from build123d import *

# Parameters (mm, degrees)
EXTRUDE_1_DEPTH        = 5
EXTRUDE_2_DEPTH        = 5
SKETCH_5_R             = 2.15
CUT_EXTRUDE_3_DEPTH    = 3.5
CUT_EXTRUDE_4_DEPTH    = 5
SKETCH_8_R             = 1.5
CUT_EXTRUDE_5_DEPTH    = 5
FILLET_1_R             = 2
FILLET_2_R             = 0.4
FILLET_4_R             = 2
FILLET_1_OF_MIRROR_2_R = 2
FILLET_2_OF_MIRROR_2_R = 0.4
FILLET_4_OF_MIRROR_2_R = 2
FILLET_3_R             = 2
SKETCH_10_R            = 0.8
CUT_EXTRUDE_6_DEPTH    = 10


with BuildPart() as part:
    # 草图2 → 凸台-拉伸1 (new body)
    with BuildSketch(Plane(origin=(0, 0, 0), x_dir=(1, 0, 0), z_dir=(0, 1, 0))):
        Polygon((0, -7.5), (0, 7.5), (-10.392304845, 13.5), (-18.392304845, 13.5), (-23.898712869, 11.116835995), (-104.216362147, 40.350069618), (-106.3513241, 34.484309861), (-103.323886643, 32.974885226), (-14.177346707, -11.471940008), (-9.177346707, -11.471940008), align=None)
    extrude_1 = extrude(amount=EXTRUDE_1_DEPTH)

    # 草图4 → 凸台-拉伸2 (add)
    with BuildSketch(Plane(origin=(0, 0, 0), x_dir=(1, 0, 0), z_dir=(0, 1, 0))):
        Polygon((-105.836537935, 43.651722154), (-104.216362147, 40.350069618), (-106.3513241, 34.484309861), (-109.577310483, 32.862960495), (-117.227960723, 33.920942119), (-119.716156877, 42.421286113), (-112.5, 47.556853078), align=None)
    extrude_2 = extrude(amount=EXTRUDE_2_DEPTH)

    # 草图5 → 切除-拉伸3 (cut)
    with BuildSketch(Plane(origin=(0, 5, 0), x_dir=(1, 0, 0), z_dir=(0, 1, 0))):
        with Locations((-112.5, 40)):
            Circle(SKETCH_5_R)
    cut_extrude_3 = extrude(amount=-CUT_EXTRUDE_3_DEPTH, mode=Mode.SUBTRACT)

    # 草图6 → 切除-拉伸4 (cut)
    with BuildSketch(Plane(origin=(0, 5, 0), x_dir=(1, 0, 0), z_dir=(0, 1, 0))):
        Polygon((-25.538029788, 4.822447994), (-66.670701963, 21.893639642), (-67.092623285, 21.03753444), (-17.588673353, -4.985970004), (-11.588673353, -4.985970004), (-7, -3), (-7, 0), (-7, 5), (-12.196152423, 8), (-18.196152423, 8), align=None)
    cut_extrude_4 = extrude(amount=-CUT_EXTRUDE_4_DEPTH, mode=Mode.SUBTRACT)

    # 草图8 → 切除-拉伸5 (cut)
    with BuildSketch(Plane(origin=(0, 5, 0), x_dir=(1, 0, 0), z_dir=(0, 1, 0))):
        with Locations((0, 4)):
            Circle(SKETCH_8_R)
        with Locations((-10, -8)):
            Circle(SKETCH_8_R)
        with Locations((-27, 9)):
            Circle(SKETCH_8_R)
    cut_extrude_5 = extrude(amount=-CUT_EXTRUDE_5_DEPTH, mode=Mode.SUBTRACT)

    # 圆角1
    fillet_1_edges = [part.edges().sort_by_distance(p)[0] for p in [
        (-23.898712869, 2.5, -11.116835995),
        (-18.196152423, 2.5, -8),
        (-12.196152423, 2.5, -8),
        (-7, 2.5, -5),
        (-7, 2.5, 3),
        (-11.588673353, 2.5, 4.985970004),
        (-17.588673353, 2.5, 4.985970004),
    ]]
    fillet(fillet_1_edges, radius=FILLET_1_R)

    # 圆角2
    fillet_2_edges = [part.edges().sort_by_distance(p)[0] for p in [
        (-67.092623285, 2.5, -21.03753444),
        (-66.670701963, 2.5, -21.893639642),
    ]]
    fillet(fillet_2_edges, radius=FILLET_2_R)

    # 圆角4
    fillet_4_edges = [part.edges().sort_by_distance(p)[0] for p in [
        (-106.3513241, 2.5, -34.484309861),
        (-104.216362147, 2.5, -40.350069618),
    ]]
    fillet(fillet_4_edges, radius=FILLET_4_R)

    # 镜向2: 凸台-拉伸1, 凸台-拉伸2, 切除-拉伸3, 切除-拉伸4, 切除-拉伸5 across Right Plane
    add(extrude_1.mirror(Plane(origin=(0, 0, 0), x_dir=(0, 0, -1), z_dir=(1, 0, 0))))
    add(extrude_2.mirror(Plane(origin=(0, 0, 0), x_dir=(0, 0, -1), z_dir=(1, 0, 0))))
    add(cut_extrude_3.mirror(Plane(origin=(0, 0, 0), x_dir=(0, 0, -1), z_dir=(1, 0, 0))), mode=Mode.SUBTRACT)
    add(cut_extrude_4.mirror(Plane(origin=(0, 0, 0), x_dir=(0, 0, -1), z_dir=(1, 0, 0))), mode=Mode.SUBTRACT)
    add(cut_extrude_5.mirror(Plane(origin=(0, 0, 0), x_dir=(0, 0, -1), z_dir=(1, 0, 0))), mode=Mode.SUBTRACT)

    # 圆角1 of 镜向2
    fillet_1_of_mirror_2_edges = [part.edges().sort_by_distance(p)[0] for p in [
        (23.898712869, 2.5, -11.116835995),
        (18.196152423, 2.5, -8),
        (12.196152423, 2.5, -8),
        (7, 2.5, -5),
        (7, 2.5, 3),
        (11.588673353, 2.5, 4.985970004),
        (17.588673353, 2.5, 4.985970004),
    ]]
    fillet(fillet_1_of_mirror_2_edges, radius=FILLET_1_OF_MIRROR_2_R)

    # 圆角2 of 镜向2
    fillet_2_of_mirror_2_edges = [part.edges().sort_by_distance(p)[0] for p in [
        (67.092623285, 2.5, -21.03753444),
        (66.670701963, 2.5, -21.893639642),
    ]]
    fillet(fillet_2_of_mirror_2_edges, radius=FILLET_2_OF_MIRROR_2_R)

    # 圆角4 of 镜向2
    fillet_4_of_mirror_2_edges = [part.edges().sort_by_distance(p)[0] for p in [
        (106.3513241, 2.5, -34.484309861),
        (104.216362147, 2.5, -40.350069618),
    ]]
    fillet(fillet_4_of_mirror_2_edges, radius=FILLET_4_OF_MIRROR_2_R)

    # 圆角3
    fillet_3_edges = [part.edges().sort_by_distance(p)[0] for p in [
        (0, 2.5, -7.5),
        (0, 2.5, 7.5),
    ]]
    fillet(fillet_3_edges, radius=FILLET_3_R)

    # 草图10 → 切除-拉伸6 (cut)
    with BuildSketch(Plane(origin=(0, 1.5, 0), x_dir=(1, 0, 0), z_dir=(0, 1, 0))):
        with Locations((-112.5, 40)):
            Circle(SKETCH_10_R)
        with Locations((112.5, 40)):
            Circle(SKETCH_10_R)
    extrude(amount=-CUT_EXTRUDE_6_DEPTH, mode=Mode.SUBTRACT)


solid = part.part
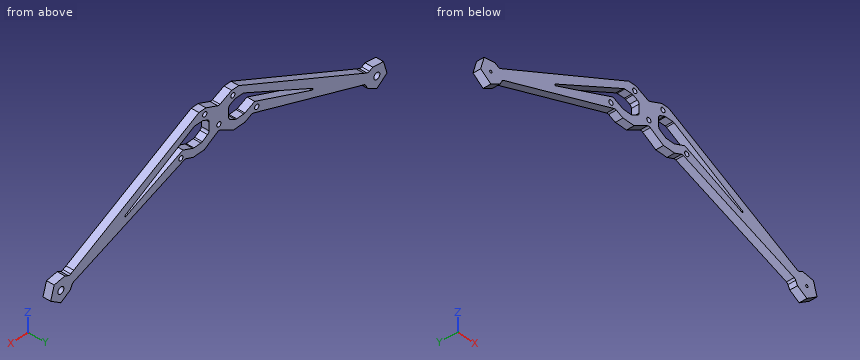
Build history of the part. All positions in model axes, mm. Round coordinates to 2 decimals unless told otherwise and drop trailing zeros. Loops run counter-clockwise (first coordinate to the right, second up) from the corner with the lowest first, then second, coordinate; pieces in that order, holes last. Notation, with made-up numbers: (-14.75, 47.25) -> (3.25, 47.25) arc R27 cw to (3.25, 84.25) -> close; hole circle Ø7 at (10.25, 29.25). An arc over 180 degrees is marked (long way). Use CSV: the item, a comma, the result in double quotes. Start each with the question number.
Q1. Saw through at B-B on z = -24. Give the cut face in (x, y), and give its area (3 significant figures).
Q2. Saw through at A-A on x = 38. Give the cut face in (y, z), and give its area (3 significant figures).
Q3. Flat gauge pins, fed straight in: pin 1 Ø1 at (x, y) = (-84, 1) entering from -Z; pin 2 Ø2 at (x, z) = (-112.5, -41) entering from +Y; pin 3 Ø2.5 at (x, y) = (-13, 2) entering from -Z; pin 4 Ø1 at (x, z) = (-112.5, -40) entering from +Y. Where does each tip first touch, or does it go through?
Q4. Saw through at D-D on x = -92. Give the cut face in (y, z), and give its area (3 significant figures).
Q5. Drill centre lines: L1, parallel to X at y = 2.45, z = -9; L2, parallel to X at y = 1.3, z = 3; L3, parallel to Z at x = 27.5, y = 1.7. Where is each one in solid material? Low to high.
Q6. Saw through at C-C on y = 3.85. Count the separate pieces of the cut face and the enclosed holes in it, and give its area (3 significant figures).
Solutions:
1,outline,"(-85.32, 0) -> (-59.29, 0) -> (-59.29, 5) -> (-85.32, 5) -> close; (59.29, 0) -> (85.32, 0) -> (85.32, 5) -> (59.29, 5) -> close"
1,area,"260 mm^2"
2,outline,"(0, -16.25) -> (5, -16.25) -> (5, -9.99) -> (0, -9.99) -> close; (0, -5.74) -> (5, -5.74) -> (5, -0.41) -> (0, -0.41) -> close"
2,area,"58.0 mm^2"
3,pin 1,"stops at z = -33.17"
3,pin 2,"stops at y = 1.5"
3,pin 3,"stops at z = -13.5"
3,pin 4,"passes through"
4,outline,"(0, -35.9) -> (5, -35.9) -> (5, -27.33) -> (0, -27.33) -> close"
4,area,"42.9 mm^2"
5,L1,"x = -55.24 to -44.19, -35.6 to -28.5, -25.5 to -2.6, 2.6 to 25.5, 28.5 to 35.6, 44.19 to 55.24"
5,L2,"x = -31.17 to -21.37, -7.49 to 7.49, 21.37 to 31.17"
5,L3,"z = -12.43 to -10.41, -7.59 to -5.64, -0.22 to 4.83"
6,separate pieces,"1"
6,enclosed holes,"9"
6,area,"2,610 mm^2"
